from build123d import *

# Parameters (mm, degrees)
SKETCH1_R                = 13
BOSS_EXTRUDE1_DEPTH      = 20
BOSS_EXTRUDE2_DEPTH      = 14
BOSS_EXTRUDE2_DEPTH_BACK = 34
SKETCH2_W                = 50
SKETCH2_H                = 14


with BuildPart() as part:
    # Sketch1 → Boss-Extrude1 (new body)
    with BuildSketch(Plane(origin=(30.485241984, 0, 0), x_dir=(0, 0, -1), z_dir=(1, 0, 0))):
        with BuildLine():
            ThreePointArc((-45.730813467, -2.952037332), (-43.709327628, -4.244029096), (-41.395669142, -4.878562094))
            ThreePointArc((-41.395669142, -4.878562094), (-41.423479526, -5.864733686), (-41.395669142, -6.850905277))
            ThreePointArc((-41.395669142, -6.850905277), (-43.709327628, -7.485438275), (-45.730813467, -8.777430039))
            ThreePointArc((-45.730813467, -8.777430039), (-45.653623019, -9.306291917), (-45.56360819, -9.833122612))
            ThreePointArc((-45.56360819, -9.833122612), (-43.241813498, -10.43720632), (-40.845312039, -10.325723271))
            ThreePointArc((-40.845312039, -10.325723271), (-40.567017505, -11.27222207), (-40.235824477, -12.201533107))
            ThreePointArc((-40.235824477, -12.201533107), (-42.240162977, -13.519969641), (-43.763462845, -15.373400306))
            ThreePointArc((-43.763462845, -15.373400306), (-43.526623058, -15.85252468), (-43.278214231, -16.325754333))
            ThreePointArc((-43.278214231, -16.325754333), (-40.883384128, -16.182798063), (-38.638625955, -15.336211705))
            ThreePointArc((-38.638625955, -15.336211705), (-38.081467911, -16.150387816), (-37.47931172, -16.931870859))
            ThreePointArc((-37.47931172, -16.931870859), (-38.978131616, -18.805153175), (-39.854134309, -21.038596032))
            ThreePointArc((-39.854134309, -21.038596032), (-39.480828712, -21.421082872), (-39.098341873, -21.794388468))
            ThreePointArc((-39.098341873, -21.794388468), (-36.864899015, -20.918385775), (-34.991616699, -19.419565879))
            ThreePointArc((-34.991616699, -19.419565879), (-34.210133656, -20.02172207), (-33.395957546, -20.578880114))
            ThreePointArc((-33.395957546, -20.578880114), (-34.242543904, -22.823638287), (-34.385500174, -25.21846839))
            ThreePointArc((-34.385500174, -25.21846839), (-33.91227052, -25.466877218), (-33.433146146, -25.703717004))
            ThreePointArc((-33.433146146, -25.703717004), (-31.579715481, -24.180417136), (-30.261278947, -22.176078636))
            ThreePointArc((-30.261278947, -22.176078636), (-29.331967911, -22.507271664), (-28.385469111, -22.785566198))
            ThreePointArc((-28.385469111, -22.785566198), (-28.49695216, -25.182067658), (-27.892868452, -27.50386235))
            ThreePointArc((-27.892868452, -27.50386235), (-27.366037757, -27.593877179), (-26.83717588, -27.671067627))
            ThreePointArc((-26.83717588, -27.671067627), (-25.545184115, -25.649581788), (-24.910651117, -23.335923302))
            ThreePointArc((-24.910651117, -23.335923302), (-23.924479526, -23.363733686), (-22.938307935, -23.335923302))
            ThreePointArc((-22.938307935, -23.335923302), (-22.303774937, -25.649581788), (-21.011783173, -27.671067627))
            ThreePointArc((-21.011783173, -27.671067627), (-20.482921295, -27.593877179), (-19.9560906, -27.50386235))
            ThreePointArc((-19.9560906, -27.50386235), (-19.352006892, -25.182067658), (-19.463489941, -22.785566198))
            ThreePointArc((-19.463489941, -22.785566198), (-18.516991142, -22.507271664), (-17.587680105, -22.176078636))
            ThreePointArc((-17.587680105, -22.176078636), (-16.269243571, -24.180417136), (-14.415812906, -25.703717004))
            ThreePointArc((-14.415812906, -25.703717004), (-13.936688532, -25.466877218), (-13.463458878, -25.21846839))
            ThreePointArc((-13.463458878, -25.21846839), (-13.606415149, -22.823638287), (-14.453001507, -20.578880114))
            ThreePointArc((-14.453001507, -20.578880114), (-13.638825396, -20.02172207), (-12.857342353, -19.419565879))
            ThreePointArc((-12.857342353, -19.419565879), (-10.984060037, -20.918385775), (-8.75061718, -21.794388468))
            ThreePointArc((-8.75061718, -21.794388468), (-8.36813034, -21.421082872), (-7.994824744, -21.038596032))
            ThreePointArc((-7.994824744, -21.038596032), (-8.870827436, -18.805153175), (-10.369647333, -16.931870859))
            ThreePointArc((-10.369647333, -16.931870859), (-9.767491142, -16.150387816), (-9.210333097, -15.336211705))
            ThreePointArc((-9.210333097, -15.336211705), (-6.965574925, -16.182798063), (-4.570744822, -16.325754333))
            ThreePointArc((-4.570744822, -16.325754333), (-4.322335994, -15.85252468), (-4.085496208, -15.373400306))
            ThreePointArc((-4.085496208, -15.373400306), (-5.608796076, -13.519969641), (-7.613134576, -12.201533107))
            ThreePointArc((-7.613134576, -12.201533107), (-7.281941548, -11.27222207), (-7.003647014, -10.325723271))
            ThreePointArc((-7.003647014, -10.325723271), (-4.607145554, -10.43720632), (-2.285350862, -9.833122612))
            ThreePointArc((-2.285350862, -9.833122612), (-2.195336033, -9.306291917), (-2.118145585, -8.777430039))
            ThreePointArc((-2.118145585, -8.777430039), (-4.139631424, -7.485438275), (-6.45328991, -6.850905277))
            ThreePointArc((-6.45328991, -6.850905277), (-6.425479526, -5.864733686), (-6.45328991, -4.878562094))
            ThreePointArc((-6.45328991, -4.878562094), (-4.139631424, -4.244029096), (-2.118145585, -2.952037332))
            ThreePointArc((-2.118145585, -2.952037332), (-2.195336033, -2.423175455), (-2.285350862, -1.89634476))
            ThreePointArc((-2.285350862, -1.89634476), (-4.607145554, -1.292261052), (-7.003647014, -1.403744101))
            ThreePointArc((-7.003647014, -1.403744101), (-7.281941548, -0.457245301), (-7.613134576, 0.472065736))
            ThreePointArc((-7.613134576, 0.472065736), (-5.608796076, 1.79050227), (-4.085496208, 3.643932934))
            ThreePointArc((-4.085496208, 3.643932934), (-4.322335994, 4.123057309), (-4.570744822, 4.596286962))
            ThreePointArc((-4.570744822, 4.596286962), (-6.965574925, 4.453330692), (-9.210333097, 3.606744334))
            ThreePointArc((-9.210333097, 3.606744334), (-9.767491142, 4.420920444), (-10.369647333, 5.202403487))
            ThreePointArc((-10.369647333, 5.202403487), (-8.870827436, 7.075685803), (-7.994824744, 9.309128661))
            ThreePointArc((-7.994824744, 9.309128661), (-8.36813034, 9.6916155), (-8.75061718, 10.064921097))
            ThreePointArc((-8.75061718, 10.064921097), (-10.984060037, 9.188918404), (-12.857342353, 7.690098508))
            ThreePointArc((-12.857342353, 7.690098508), (-13.638825396, 8.292254699), (-14.453001507, 8.849412743))
            ThreePointArc((-14.453001507, 8.849412743), (-13.606415149, 11.094170916), (-13.463458878, 13.489001019))
            ThreePointArc((-13.463458878, 13.489001019), (-13.936688532, 13.737409846), (-14.415812906, 13.974249633))
            ThreePointArc((-14.415812906, 13.974249633), (-16.269243571, 12.450949765), (-17.587680105, 10.446611265))
            ThreePointArc((-17.587680105, 10.446611265), (-18.516991142, 10.777804293), (-19.463489941, 11.056098827))
            ThreePointArc((-19.463489941, 11.056098827), (-19.352006892, 13.452600287), (-19.9560906, 15.774394978))
            ThreePointArc((-19.9560906, 15.774394978), (-20.482921295, 15.864409807), (-21.011783173, 15.941600255))
            ThreePointArc((-21.011783173, 15.941600255), (-22.303774937, 13.920114416), (-22.938307935, 11.60645593))
            ThreePointArc((-22.938307935, 11.60645593), (-23.924479526, 11.634266314), (-24.910651117, 11.60645593))
            ThreePointArc((-24.910651117, 11.60645593), (-25.545184115, 13.920114416), (-26.83717588, 15.941600255))
            ThreePointArc((-26.83717588, 15.941600255), (-27.366037757, 15.864409807), (-27.892868452, 15.774394978))
            ThreePointArc((-27.892868452, 15.774394978), (-28.49695216, 13.452600287), (-28.385469111, 11.056098827))
            ThreePointArc((-28.385469111, 11.056098827), (-29.331967911, 10.777804293), (-30.261278947, 10.446611265))
            ThreePointArc((-30.261278947, 10.446611265), (-31.579715481, 12.450949765), (-33.433146146, 13.974249633))
            ThreePointArc((-33.433146146, 13.974249633), (-33.91227052, 13.737409846), (-34.385500174, 13.489001019))
            ThreePointArc((-34.385500174, 13.489001019), (-34.242543904, 11.094170916), (-33.395957546, 8.849412743))
            ThreePointArc((-33.395957546, 8.849412743), (-34.210133656, 8.292254699), (-34.991616699, 7.690098508))
            ThreePointArc((-34.991616699, 7.690098508), (-36.864899015, 9.188918404), (-39.098341873, 10.064921097))
            ThreePointArc((-39.098341873, 10.064921097), (-39.480828712, 9.6916155), (-39.854134309, 9.309128661))
            ThreePointArc((-39.854134309, 9.309128661), (-38.978131616, 7.075685803), (-37.47931172, 5.202403487))
            ThreePointArc((-37.47931172, 5.202403487), (-38.081467911, 4.420920444), (-38.638625955, 3.606744334))
            ThreePointArc((-38.638625955, 3.606744334), (-40.883384128, 4.453330692), (-43.278214231, 4.596286962))
            ThreePointArc((-43.278214231, 4.596286962), (-43.526623058, 4.123057309), (-43.763462845, 3.643932934))
            ThreePointArc((-43.763462845, 3.643932934), (-42.240162977, 1.79050227), (-40.235824477, 0.472065736))
            ThreePointArc((-40.235824477, 0.472065736), (-40.567017505, -0.457245301), (-40.845312039, -1.403744101))
            ThreePointArc((-40.845312039, -1.403744101), (-43.241813498, -1.292261052), (-45.56360819, -1.89634476))
            ThreePointArc((-45.56360819, -1.89634476), (-45.653623019, -2.423175455), (-45.730813467, -2.952037332))
        make_face()
        with Locations(Location((-23.924479526, -5.864733686, 0), (0, 0, 180))):
            Circle(SKETCH1_R, mode=Mode.SUBTRACT)
    extrude(amount=-BOSS_EXTRUDE1_DEPTH)

    # Sketch2 → Boss-Extrude2 (add, two sides: drawn at the far end of the back side and taken through both)
    with BuildSketch(Plane(origin=(30.485241984, 0, 0), x_dir=(0, 0, -1), z_dir=(1, 0, 0)).offset(-BOSS_EXTRUDE2_DEPTH_BACK)):
        with Locations((-24.233465749, 14.653188973)):
            Rectangle(SKETCH2_W, SKETCH2_H)
    extrude(amount=BOSS_EXTRUDE2_DEPTH + BOSS_EXTRUDE2_DEPTH_BACK)


solid = part.part
The model under review builds one solid part; all positions refer to its coordinate system, in mm. A direction names the side the tool comes from. Give positions to 0.01 mm unless a question says otherwise; leave off trailing zeros. Write each loop counter-clockwise with the first axis right and the second up, starting at its lowest first coordinate (ties: lowest second). Pieces come first, ordered by that corner, then holes.
1. Wall thickness on L1, parallel to Z at x = 23.5, y = -20.5; L2, parallel to Y at x = 16.5, z = 10; L3, parallel to Y at x = 33, z = 11: over which ranges is each line inside the solid? List them lowest first.
2. Add section D-D, the plane z = 31. Write out the cut boundary in (x, y).
3. For P1, Ø5, axis at y = -19.5, z = 35.5, coming from the -X side; P2, Ø3, axis at y = -7.5, z = 43, coming from the +X side, all flat-tipped, find the tip position at first contact; note any pin that passes through.
4. Add section A-A, the plane y = 2.5. Write out the cut boundary in (x, z).
5. Add section B-B, the plane z = 12. Write out the cut boundary in (x, y).
6. Add section C-C, the plane x = 35. Write out the cut boundary in (y, z).
7. Draft analysis for pull direction Y (two halves, no side actions). For faces 1 (the cylindrical face through (20.63, -11.26, 40.57)), 2 (the cylindrical face through (20.6, -24.2, 31.6)), 3 (the cylindrical face through (20.63, -4.23, 43.74)), 4 (the flat face through (10.485, -19, 22)), state which applies: +Y half, -Y half, draft (parallel to the pull), parting line (faces both ways), or undercut.
8. Tool access review of faces 5 (the cylindrical face through (20.63, -13.5, 42.22)), 6 (the flat face through (30.485, -19, 22)), 7 (the cylindrical face through (20.6, 1.8, 5.6)), 8 (the cylindrical face through (20.625, -22.791, 34.235)): name each direction out of +Z, -Z, +X, -X, +Y, -Y from which nothing blocks a thin tool from reaching the whole face with its end or side.
Worked answers:
1. L1: z = 8.14 to 11.63, 14.33 to 33.52, 36.22 to 39.71
1. L2: y = -21.4 to -17.3, -16.46 to 4.73, 5.57 to 21.65
1. L3: y = 7.65 to 21.65
2. outline: (-3.51, 7.65) - (10.49, 7.65) - (10.49, 5.04) - (30.49, 5.04) - (30.49, 7.65) - (44.49, 7.65) - (44.49, 21.65) - (-3.51, 21.65) - close; (10.49, -23.46) - (30.49, -23.46) - (30.49, -16.77) - (10.49, -16.77) - close
3. P1: stops at x = 10.49
3. P2: stops at x = 30.49
4. outline: (10.49, 4.91) - (30.49, 4.91) - (30.49, 13.97) - (10.49, 13.97) - close; (10.49, 33.88) - (30.49, 33.88) - (30.49, 42.94) - (10.49, 42.94) - close
5. outline: (-3.51, 7.65) - (10.49, 7.65) - (10.49, -0.69) - (30.49, -0.69) - (30.49, 7.65) - (44.49, 7.65) - (44.49, 21.65) - (-3.51, 21.65) - close; (10.49, -20.22) - (30.49, -20.22) - (30.49, -11.04) - (10.49, -11.04) - close
6. outline: (7.65, -0.77) - (21.65, -0.77) - (21.65, 49.23) - (7.65, 49.23) - close
7. face 1: undercut
7. face 2: -Y half
7. face 3: undercut
7. face 4: draft
8. face 5: +Z, +X, -X
8. face 6: +Z, -Z, +X, -Y
8. face 7: -Z, +X, -X
8. face 8: +X, -X
